```python
from build123d import *

# Parameters (mm, degrees)
F1_DEPTH = 40
F3_R     = 7.5
F4_DEPTH = 45


with BuildPart() as f1:
    # F0 (on Front) → F1 (new body)
    with BuildSketch(Plane.XZ):
        with BuildLine():
            Line((-34.882351, 15.875), (-34.882351, 2.875))
            ThreePointArc((-34.882351, 2.875), (-34.589458, 2.167893), (-33.882351, 1.875))
            Line((-33.882351, 1.875), (-15.73958, 1.875))
            ThreePointArc((-15.73958, 1.875), (-15.099145, 2.106987), (-14.755856, 2.695313))
            ThreePointArc((-14.755856, 2.695313), (1.353174, 14.938839), (15, 0))
            Line((15, 0), (22.5, 0))
            ThreePointArc((22.5, 0), (9.4235, 20.431536), (-14.606458, 17.114362))
            ThreePointArc((-14.606458, 17.114362), (-14.909685, 16.936747), (-15.255634, 16.875))
            Line((-15.255634, 16.875), (-33.882351, 16.875))
            ThreePointArc((-33.882351, 16.875), (-34.589458, 16.582107), (-34.882351, 15.875))
        make_face()
    extrude(amount=F1_DEPTH)

    # F2: F1 across face


with BuildPart() as f1_1:
    add(f1.part)
    add(f1.part.mirror(Plane(origin=(18.75, -20, 0), x_dir=(1, 0, 0), z_dir=(0, 0, -1))))

    # F3 (on face) → F4 (cut)
    with BuildSketch(Plane.XY.offset(16.875)):
        with Locations((-23.382351, -20)):
            Circle(F3_R)
    extrude(amount=-F4_DEPTH, mode=Mode.SUBTRACT)


solid = f1_1.part
```
Check sheet for the modelled part. Datum: model origin and axes. Units: mm. A direction names the side the tool comes from. Give positions to 0.01 mm unless a question says otherwise; leave off trailing zeros. Loops run counter-clockwise (first coordinate to the right, second up) from the corner with the lowest first, then second, coordinate; pieces in that order, holes last. Notation, with made-up numbers: M -3.75,71 L 44.25,71 A28 ccw 44.25,101 Z; hole C -40,32 d6. An arc over 180 degrees is marked long. Answer as CSV lines item,"result".
Item 1: Sectioned sample at B-B, the plane x = -6.5. Enter the section's corners in (y, z).
Reply:
outline,"M -40,-21.54 L 0,-21.54 L 0,-13.52 L -40,-13.52 Z; M -40,13.52 L 0,13.52 L 0,21.54 L -40,21.54 Z"
Item 2: Set-up check for faces 1 (the face through (-31, -15, -1.875)), 2 (the face through (-31, -15, 16.875)), 3 (the face through (-31, -15, -16.875)): record each of +Z, -Z, +X, -X, +Y, -Y from which the full face is reachable in a straight line by a thin tool's end or side.
Reply:
face 1,"-X, +Y, -Y"
face 2,"+Z, -X, +Y, -Y"
face 3,"-Z, -X, +Y, -Y"
Item 3: Scan lines: L1, parallel to Z at x = -29, y = -13 (3 decimals); L2, parallel to Z at x = 0.5, y = -34.5; L3, parallel to X at y = -17, z = 12.5. Record each from-to range of solid material in increasing order.
Reply:
L1,"-16.875 to -1.875, 1.875 to 16.875"
L2,"-22.49 to -14.99, 14.99 to 22.49"
L3,"-34.88 to -30.26, -16.51 to -8.29, 8.29 to 18.71"
Item 4: Depth check by flat-ended pin: pin 1 Ø5.5 at (x, y) = (-25, -17) entering from -Z; pin 2 Ø5 at (x, y) = (-8, -23.5) entering from -Z; pin 3 Ø3 at (x, y) = (-4, -8.5) entering from -Z; pin 4 Ø20 at (x, y) = (-25.5, -16.5) entering from +Z (3 decimals). Enter the tip coordinate at first touch or a pass-through.
Reply:
pin 1,"through"
pin 2,"z = -21.82"
pin 3,"z = -22.36"
pin 4,"z = 16.875"
Item 5: Sectioned sample at C-C, the plane y = -20. Enter the section's corners in (x, z) (3 decimals).
Reply:
outline,"M -34.882,-15.875 A1 ccw -33.882,-16.875 L -30.882,-16.875 L -30.882,-1.875 L -33.882,-1.875 A1 ccw -34.882,-2.875 Z; M -34.882,2.875 A1 ccw -33.882,1.875 L -30.882,1.875 L -30.882,16.875 L -33.882,16.875 A1 ccw -34.882,15.875 Z; M -15.882,-16.875 L -15.256,-16.875 A1 cw -14.606,-17.114 A22.5 ccw 22.5,0 A22.5 ccw -14.606,17.114 A1 cw -15.256,16.875 L -15.882,16.875 L -15.882,1.875 L -15.74,1.875 A1 ccw -14.756,2.695 A15 cw long -14.756,-2.695 A1 ccw -15.74,-1.875 L -15.882,-1.875 Z"
Item 6: Sectioned sample at A-A, the plane z = 10.5. Enter the section's corners in (x, y), then the cut area to 3 significant figures.
Reply:
outline,"M -34.88,-40 L -10.71,-40 L -10.71,0 L -34.88,0 Z; M 10.71,-40 L 19.9,-40 L 19.9,0 L 10.71,0 Z; hole C -23.38,-20 d15"
area,"1,160 mm^2"
Item 7: Sectioned sample at D-D, the plane y = -31. Enter the section's corners in (x, z) (3 decimals), then the cut area to 3 significant figures.
Reply:
outline,"M -34.882,-15.875 A1 ccw -33.882,-16.875 L -15.256,-16.875 A1 cw -14.606,-17.114 A22.5 ccw 22.5,0 A22.5 ccw -14.606,17.114 A1 cw -15.256,16.875 L -33.882,16.875 A1 ccw -34.882,15.875 L -34.882,2.875 A1 ccw -33.882,1.875 L -15.74,1.875 A1 ccw -14.756,2.695 A15 cw long -14.756,-2.695 A1 ccw -15.74,-1.875 L -33.882,-1.875 A1 ccw -34.882,-2.875 Z"
area,"1,300 mm^2"
Item 8: Draft check along X on faces 4 (the face through (-28.91, -14.93, -9.27)), 5 (the face through (-34.882, -20, 9)), 6 (the face through (-31, -15, 1.875)), 7 (the face through (-28.91, -14.93, 9.48)). Enter one of: pulls with the +X half, pulls with the -X half, needs draft (parallel to the pull), parting line crosses it, or undercut.
Reply:
face 4,"undercut"
face 5,"pulls with the -X half"
face 6,"needs draft"
face 7,"undercut"
